Geometry check sheet. Reference: the model listing, model coordinates, mm. A direction names the side the tool comes from. Coordinates: 2 decimals unless noted, no trailing zeros. Loops run counter-clockwise (first coordinate to the right, second up) from the corner with the lowest first, then second, coordinate; pieces in that order, holes last. Notation, with made-up numbers: (78.25, -40) - (114.25, -40) arc R13 ccw to (114.25, -23) - close; hole circle Ø3 at (7.5, 32.5). An arc over 180 degrees is marked (long way). Write item = value, one per line. Start each with the question number.
from build123d import *

# Parameters (mm, degrees)
PAD_DEPTH = 4


with BuildPart() as part:
    # Sketch → Pad (new body)
    with BuildSketch(Plane.XY):
        with BuildLine():
            Line((0.353553, 0), (28, 0))
            ThreePointArc((28, 0), (29, 0.57735), (29, 1.732051))
            Line((29, 1.732051), (15.176777, 25.674576))
            ThreePointArc((15.176777, 25.674576), (14.962097, 25.839306), (14.693814, 25.803985))
            Line((14.693814, 25.803985), (14.007148, 25.407539))
            ThreePointArc((14.007148, 25.407539), (13.842418, 25.192859), (13.877739, 24.924576))
            Line((21.131753, 12.360254), (13.877739, 24.924576))
            ThreePointArc((21.131753, 10.960254), (21.319318, 11.660254), (21.131753, 12.360254))
            Line((21.131753, 10.960254), (16.074018, 2.2))
            ThreePointArc((14.861583, 1.5), (15.561583, 1.687564), (16.074018, 2.2))
            Line((0.353553, 1.5), (14.861583, 1.5))
            ThreePointArc((0.353553, 1.5), (0.103553, 1.396447), (0, 1.146447))
            Line((0, 1.146447), (0, 0.353553))
            ThreePointArc((0, 0.353553), (0.103553, 0.103553), (0.353553, 0))
        make_face()
        with BuildLine():
            Line((21.901924, 9.294229), (17.901924, 2.366025))
            ThreePointArc((17.901924, 2.366025), (17.901924, 1.788675), (18.401924, 1.5))
            Line((26.401924, 1.5), (18.401924, 1.5))
            ThreePointArc((26.401924, 1.5), (26.901924, 1.788675), (26.901924, 2.366025))
            Line((22.901924, 9.294229), (26.901924, 2.366025))
            ThreePointArc((22.901924, 9.294229), (22.401924, 9.582904), (21.901924, 9.294229))
        make_face(mode=Mode.SUBTRACT)
    extrude(amount=PAD_DEPTH)


solid = part.part
(1) Tool access check on faces 1 (the face through (20, 6, 2)), 2 (the face through (19, 6, 0)), 3 (the face through (15.55, 1.68, 1.97)). Record the directions out of +Z, -Z, +X, -X, +Y, -Y that give a thin tool (end or side, any length) a straight path to the whole face; none if there is none.
(2) Sectioned sample at A-A on z = 0.7. Enter the section's corners in (x, y), plus the area to 3 significant figures.
(3) Sectioned sample at D-D on x = 9. Enter the section's corners in (y, z).
(4) Draft check along X on faces 4 (the face through (17.56, 18.55, 1.97)), 5 (the face through (19, 6, 4)), 6 (the face through (28.99, 0.56, 1.97)), 7 (the face through (22.41, 9.583, 1.972)). Enter one of: pulls with the +X half, pulls with the -X half, needs draft (parallel to the pull), parting line crosses it, or undercut.
(5) Sectioned sample at C-C on x = 16.75. Enter the section's corners in (y, z).
(6) Scan lines: line 1 (Y direction, x = 19.5, z = 1.3); line 2 (Y direction, x = 6, z = 0.45); line 3 (Y direction, x = 26.5, z = 0.85). Record each from-to range of solid material in increasing order.
(7) Sectioned sample at B-B on y = 5.5. Enter the section's corners in (x, z).
(8) Depth check by flat-ended pin: pin 1 (1.5 mm diameter, centred on y = 17, z = 2, fed in from +X); pin 2 (1.2 mm diameter, centred on x = 22.5, z = 1.5, fed in from +Y); pin 3 (2 mm diameter, centred on y = 3.5, z = 1, fed in from +X). Enter the tip coordinate at first touch or a pass-through.
Working result:
q1.face_1 = +Z, -Z
q1.face_2 = -Z, +X, -X, +Y, -Y
q1.face_3 = +Z, -Z, -X
q2.outline = (0, 0.35) arc R0.35 ccw to (0.35, 0) - (28, 0) arc R1.15 ccw to (29, 1.73) - (15.18, 25.67) arc R0.35 ccw to (14.69, 25.8) - (14.01, 25.41) arc R0.35 ccw to (13.88, 24.92) - (21.13, 12.36) arc R1.4 cw to (21.13, 10.96) - (16.07, 2.2) arc R1.4 cw to (14.86, 1.5) - (0.35, 1.5) arc R0.35 ccw to (0, 1.15) - close; hole (17.9, 2.37) arc R0.58 ccw to (18.4, 1.5) - (26.4, 1.5) arc R0.58 ccw to (26.9, 2.37) - (22.9, 9.29) arc R0.58 ccw to (21.9, 9.29) - close
q2.area = 102 mm2
q3.outline = (0, 0) - (1.5, 0) - (1.5, 4) - (0, 4) - close
q4.face_4 = pulls with the -X half
q4.face_5 = needs draft
q4.face_6 = pulls with the +X half
q4.face_7 = undercut
q5.outline = (0, 0) - (3.37, 0) - (3.37, 4) - (0, 4) - close; (19.95, 0) - (22.95, 0) - (22.95, 4) - (19.95, 4) - close
q6.line_1 = 0 to 1.5, 5.13 to 8.13, 15.19 to 18.19
q6.line_2 = 0 to 1.5
q6.line_3 = 0 to 1.51, 3.06 to 6.06
q7.outline = (17.98, 0) - (19.71, 0) - (19.71, 4) - (17.98, 4) - close; (25.09, 0) - (26.82, 0) - (26.82, 4) - (25.09, 4) - close
q8.pin_1 = 20.62
q8.pin_2 = 14.03
q8.pin_3 = 28.56
